Autodesk Inventor part; units mm, degrees
ref_plane "YZ Plane" through (0, 0, 0) normal (1, 0, 0) x (0, 1, 0)
ref_plane "XZ Plane" through (0, 0, 0) normal (0, 1, 0) x (-1, 0, 0)
ref_plane "XY Plane" through (0, 0, 0) normal (0, 0, 1) x (1, 0, 0)
sketch "Sketch5" plane through (0, 0, 0) normal (0, 1, 0) x (-1, 0, 0)
  line L0 (27.9234, 26.0727) -> (-26.467, 26.0727)
  line L1 (-26.467, 26.0727) -> (-26.467, -28.3178)
  line L2 (-26.467, -28.3178) -> (27.9234, -28.3178)
  line L3 (27.9234, -28.3178) -> (27.9234, 26.0727)
  point P0 (0, 0)
extrude "Extrusion3" add sketch "Sketch5" along normal blind 6.35
sketch "Sketch6" plane through (0, 0, 0) normal (0, -1, 0) x (1, 0, 0)
  line L0 (-32.7834, 33.8762) -> (32.7834, 33.8762)
  line L1 (32.7834, 33.8762) -> (32.7834, -36.936)
  line L2 (32.7834, -36.936) -> (-32.7834, -36.936)
  line L3 (-32.7834, -36.936) -> (-32.7834, 33.8762)
  point P0 (0, 0)
extrude "Extrusion4" add sketch "Sketch6" along normal blind 6.35
sketch "Sketch7" plane through (0, 6.35, 0) normal (0, 1, 0) x (1, 0, 0)
  line L0 (-19.5244, 21.2) -> (18.7958, 21.2)
  line L1 (18.7958, 21.2) -> (18.7958, -19.5972)
  line L2 (18.7958, -19.5972) -> (-19.5244, -19.5972)
  line L3 (-19.5244, -19.5972) -> (-19.5244, 21.2)
  point P0 (0, 0)
extrude "Extrusion5" add sketch "Sketch7" along normal blind 6.35
sketch "Sketch8" plane through (0, 12.7, 0) normal (0, 1, 0) x (1, 0, 0)
  circle A0 centre (0, 0) radius 8.1896
hole "Hole1" at (0, 12.7, 0) direction (0, -1, 0) diameter 25.4 end through all
properties part number "1st part ever"
The model under review builds one solid part; all positions refer to its coordinate system, in mm. A direction names the side the tool comes from. Give positions to 0.01 mm unless a question says otherwise; leave off trailing zeros. Write each loop counter-clockwise with the first axis right and the second up, starting at its lowest first coordinate (ties: lowest second). Pieces come first, ordered by that corner, then holes. Notation, with made-up numbers: M 46.5,-9 L 96.5,-9 A35 cw 96.5,23 Z; hole C -37,23.5 d3. An arc over 180 degrees is marked long. Answer in a Markdown table with one row per item.
Item 1: Add section D-D on x = 0. Give the boundary of the cut face in (y, z).
Check sheet entries:
| item | result |
|---|---|
| outline | M -6.35,-36.94 L 0,-36.94 L 0,-28.32 L 6.35,-28.32 L 6.35,-21.2 L 12.7,-21.2 L 12.7,-12.7 L -6.35,-12.7 Z; M -6.35,12.7 L 12.7,12.7 L 12.7,19.6 L 6.35,19.6 L 6.35,26.07 L 0,26.07 L 0,33.88 L -6.35,33.88 Z |
Item 2: Add section A-A on x = -24. Give the boundary of the cut face in (y, z), plus the area to 3 significant figures.
Check sheet entries:
| item | result |
|---|---|
| outline | M -6.35,-36.94 L 0,-36.94 L 0,-28.32 L 6.35,-28.32 L 6.35,26.07 L 0,26.07 L 0,33.88 L -6.35,33.88 Z |
| area | 795 mm2 |
Item 3: Draft analysis for pull direction X (two halves, no side actions). For faces 1 (the face through (-30, 0, -1)), 2 (the face through (-19.524, 9, -1)), 3 (the face through (12.4, 3.04, -2.75)), state which applies: +X half, -X half, draft (parallel to the pull), parting line (faces both ways), or undercut.
Check sheet entries:
| item | result |
|---|---|
| face 1 | draft |
| face 2 | -X half |
| face 3 | undercut |
Item 4: For line 1 along X through (y, z) = (5.5, 0); line 2 along Z through (x, y) = (0, 8.5); line 3 along Y through (x, z) = (-29.5, -6.5), list the stretches that pass through material, from the lowest coordinate up.
Check sheet entries:
| item | result |
|---|---|
| line 1 | -27.92 to -12.7, 12.7 to 26.47 |
| line 2 | -21.2 to -12.7, 12.7 to 19.6 |
| line 3 | -6.35 to 0 |
Item 5: For P1, Ø2, axis at y = 2.5, z = 6, coming from the +X side; P2, Ø3, axis at x = -6.5, y = 9, coming from the -Z side; P3, Ø5, axis at y = 3.5, z = 6, coming from the -X side; P4, Ø7, axis at x = -5.5, y = 2.5, coming from the +Z side, all flat-tipped, find the tip position at first contact; note any pin that passes through.
Check sheet entries:
| item | result |
|---|---|
| P1 | x = 26.47 |
| P2 | z = -21.2 |
| P3 | x = -27.92 |
| P4 | z = 33.88 |
Item 6: Add section B-B on z = 0. Give the boundary of the cut face in (x, y), plus the area to 3 significant figures.
Check sheet entries:
| item | result |
|---|---|
| outline | M -32.78,-6.35 L -12.7,-6.35 L -12.7,12.7 L -19.52,12.7 L -19.52,6.35 L -27.92,6.35 L -27.92,0 L -32.78,0 Z; M 12.7,-6.35 L 32.78,-6.35 L 32.78,0 L 26.47,0 L 26.47,6.35 L 18.8,6.35 L 18.8,12.7 L 12.7,12.7 Z |
| area | 521 mm2 |
Item 7: Tool access review of faces 4 (the face through (0, 3, -28.318)), 5 (the face through (-27.923, 3, -2)), 6 (the face through (18.796, 9, -1)), 7 (the face through (-32.783, -3, -2)), 8 (the face through (0, 9, 19.597)): name each direction out of +Z, -Z, +X, -X, +Y, -Y from which nothing blocks a thin tool from reaching the whole face with its end or side.
Check sheet entries:
| item | result |
|---|---|
| face 4 | -Z, +X, -X, +Y |
| face 5 | +Z, -Z, -X, +Y |
| face 6 | +Z, -Z, +X, +Y |
| face 7 | +Z, -Z, -X, +Y, -Y |
| face 8 | +Z, +X, -X, +Y |
Item 8: Add section C-C on y = -1. Give the boundary of the cut face in (x, z), plus the area to 3 significant figures.
Check sheet entries:
| item | result |
|---|---|
| outline | M -32.78,-36.94 L 32.78,-36.94 L 32.78,33.88 L -32.78,33.88 Z; hole C 0,0 d25.4 |
| area | 4,140 mm2 |
